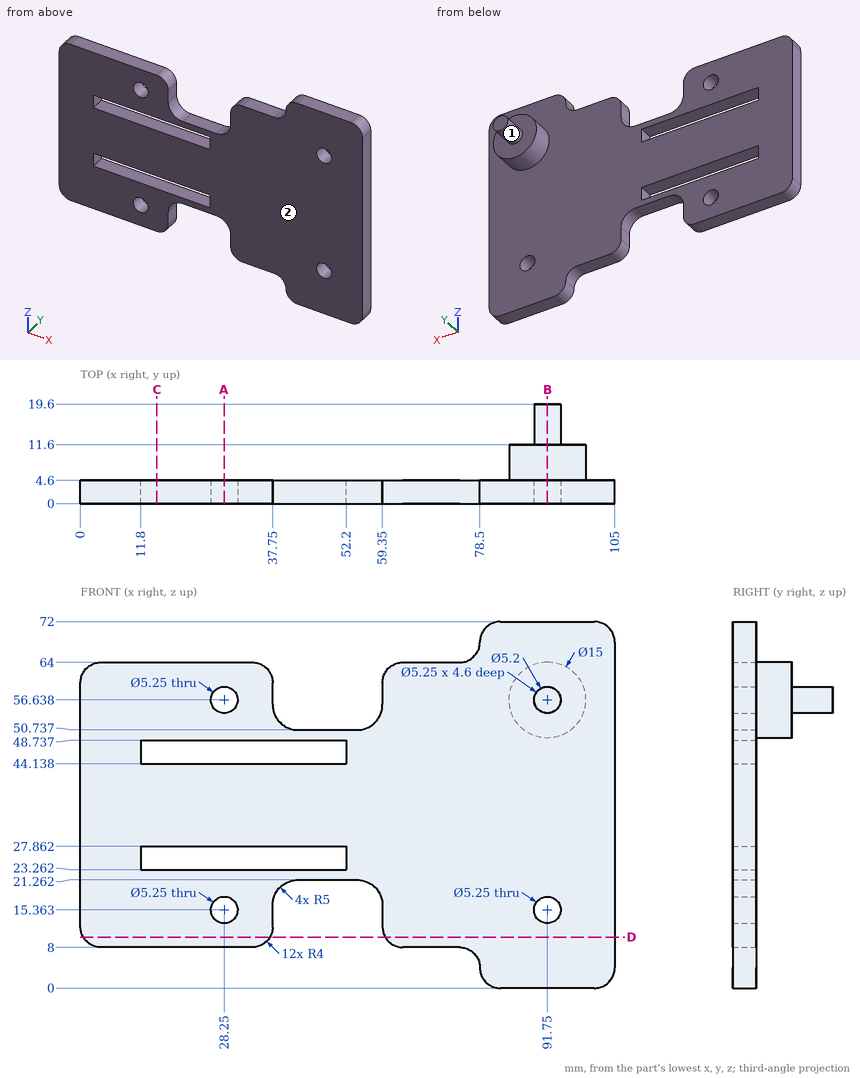
Geometry: see drawing. Coordinates: mm, zero at the bounding-box minimum. A direction names the side the tool comes from. Give positions to 0.01 mm unless a question says otherwise; leave off trailing zeros. Loops run counter-clockwise (first coordinate to the right, second up) from the corner with the lowest first, then second, coordinate; pieces in that order, holes last. Notation, with made-up numbers: M 4,-18.75 L 61,-18.75 A18 ccw 61,4.25 Z; hole C 89,60 d1. An arc over 180 degrees is marked long. Answer as CSV lines item,"result". Start each with the question number.
1. Pin query (flat end, axial travel): P1, Ø4, axis at x = 28.25, z = 15.36, coming from the -Y side; P2, Ø5, axis at x = 25, y = 3.5, coming from the +Z side; P3, Ø3.5, axis at x = 46.5, y = 3.5, coming from the +Z side; P4, Ø3.5, axis at x = 21, y = 3, coming from the -Z side. Return the tip coordinate at first contact, or that it passes through.
2. Section C-C on x = 15. Return loops of the section in (y, z).
3. Section B-B on x = 91.75. Return loops of the section in (y, z).
4. Line query: L1, parallel to Z at x = 91.75, y = 2.8; L2, parallel to X at y = 4, z = 17 (1 decimal); L3, parallel to X at y = 17.75, z = 57 (1 decimal). Output: solid intervals per line, ascending.
5. Section A-A on x = 28.25. Return loops of the section in (y, z), plus the area to 3 significant figures.
6. Section D-D on z = 10. Return loops of the section in (x, y) (1 decimal).
7. Reachability of the marked faces 1 and 2 from +Z, -Z, +X, -X, +Y, -Y: full face, straight path, thin tool, end or side. Return the list, or none.
Computed values:
1,P1,"passes through"
1,P2,"stops at z = 64"
1,P3,"stops at z = 50.74"
1,P4,"stops at z = 8"
2,outline,"M 0,8 L 4.6,8 L 4.6,23.26 L 0,23.26 Z; M 0,27.86 L 4.6,27.86 L 4.6,44.14 L 0,44.14 Z; M 0,48.74 L 4.6,48.74 L 4.6,64 L 0,64 Z"
3,outline,"M 0,0 L 4.6,0 L 4.6,12.74 L 0,12.74 Z; M 0,17.99 L 4.6,17.99 L 4.6,49.14 L 11.6,49.14 L 11.6,54.04 L 19.6,54.04 L 19.6,59.24 L 11.6,59.24 L 11.6,64.14 L 4.6,64.14 L 4.6,72 L 0,72 L 0,59.26 L 4.6,59.26 L 4.6,54.01 L 0,54.01 Z"
4,L1,"z = 0 to 12.74, 17.99 to 54.01, 59.26 to 72"
4,L2,"x = 0 to 26.2, 30.3 to 37.8, 59.3 to 89.7, 93.8 to 105"
4,L3,"x = 89.2 to 94.3"
5,outline,"M 0,8 L 4.6,8 L 4.6,12.74 L 0,12.74 Z; M 0,17.99 L 4.6,17.99 L 4.6,23.26 L 0,23.26 Z; M 0,27.86 L 4.6,27.86 L 4.6,44.14 L 0,44.14 Z; M 0,48.74 L 4.6,48.74 L 4.6,54.01 L 0,54.01 Z; M 0,59.26 L 4.6,59.26 L 4.6,64 L 0,64 Z"
5,area,"167 mm²"
6,outline,"M 0.5,0 L 37.2,0 L 37.2,4.6 L 0.5,4.6 Z; M 59.9,0 L 105,0 L 105,4.6 L 59.9,4.6 Z"
7,face 1,"+Y"
7,face 2,"+Z, -Z, +X, -X, -Y"
